The figure shows three views and two pictorial views of one solid part (mm, origin at its lowest corner). Answer the questions. Coordinates: 2 decimals unless noted, no trailing zeros. Order: outer loops, then holes, each group sorted by start corner. A loop starts at its lowest first (then second) coordinate and runs counter-clockwise, first axis right, second up. Notation, with made-up numbers: (-17.75, 46) -> (-9.75, 46) arc R26 ccw to (-9.75, 85) -> close; hole circle Ø8 at (52.25, 67.5). An arc over 180 degrees is marked (long way). Return JSON: item names as keys, results as strings.
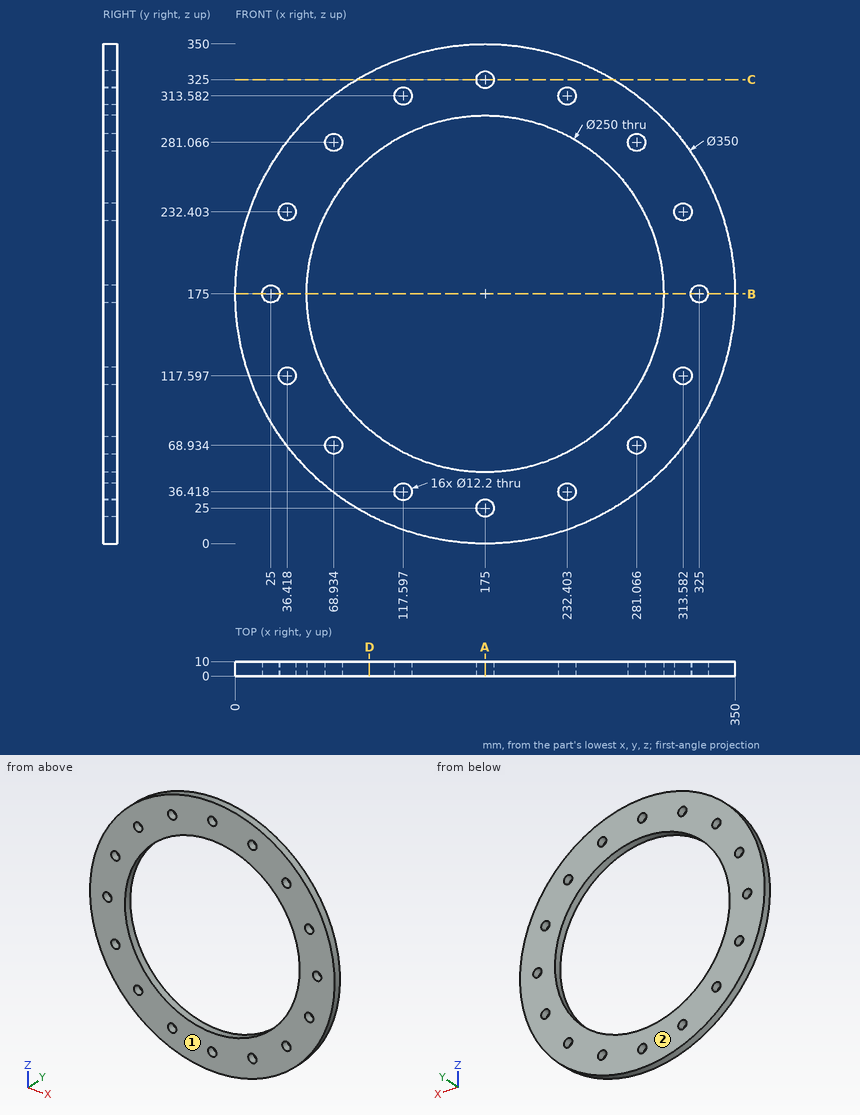
Item 1: Find the intervals of material crossed by probe 1 along X at (y, z) = (6.25, 175); probe 2 along X at (y, z) = (3.5, 170) (1 decimal); probe 3 along Z at (x, y) = (39.5, 6.75) (1 decimal), in increasing order.
Answer list:
{"probe 1": "0 to 18.9, 31.1 to 50, 300 to 318.9, 331.1 to 350", "probe 2": "0.1 to 21.5, 28.5 to 50.1, 299.9 to 321.5, 328.5 to 349.9", "probe 3": "64.3 to 112.3, 122.9 to 227.1, 237.7 to 285.7"}
Item 2: The part is cut by section C-C on z = 325. Determine the outline of the cut face in (x, y), plus the area to 3 significant figures.
Answer list:
{"outline": "(84.86, 0) -> (168.9, 0) -> (168.9, 10) -> (84.86, 10) -> close; (181.1, 0) -> (265.14, 0) -> (265.14, 10) -> (181.1, 10) -> close", "area": "1,680 mm2"}
Item 3: The part is cut by section B-B on z = 175. Determine the outline of the cut face in (x, y).
Answer list:
{"outline": "(0, 0) -> (18.9, 0) -> (18.9, 10) -> (0, 10) -> close; (31.1, 0) -> (50, 0) -> (50, 10) -> (31.1, 10) -> close; (300, 0) -> (318.9, 0) -> (318.9, 10) -> (300, 10) -> close; (331.1, 0) -> (350, 0) -> (350, 10) -> (331.1, 10) -> close"}
Item 4: Flat-ended cylindrical pins translate along their axes: pin 1 (1.5 mm diameter, centred on y = 4, z = 193.5, fed in from -X); pin 2 (5 mm diameter, centred on x = 156, y = 5.5, fed in from +Z); pin 3 (3 mm diameter, centred on y = 5, z = 310, fed in from -X). Find the tip coordinate at first contact, or state that the pin passes through.
Answer list:
{"pin 1": "x = 0.9", "pin 2": "z = 349.22", "pin 3": "x = 61.85"}
Item 5: The part is cut by section A-A on x = 175. Determine the outline of the cut face in (y, z).
Answer list:
{"outline": "(0, 0) -> (10, 0) -> (10, 18.9) -> (0, 18.9) -> close; (0, 31.1) -> (10, 31.1) -> (10, 50) -> (0, 50) -> close; (0, 300) -> (10, 300) -> (10, 318.9) -> (0, 318.9) -> close; (0, 331.1) -> (10, 331.1) -> (10, 350) -> (0, 350) -> close"}
Item 6: Determine the mould class of the marked faces 1 and 2 for opening direction Y: pulls with the +Y half, pulls with the -Y half, needs draft (parallel to the pull), parting line crosses it, or undercut.
Answer list:
{"face 1": "pulls with the -Y half", "face 2": "pulls with the +Y half"}
Item 7: The part is cut by section D-D on x = 94. Determine the outline of the cut face in (y, z) (1 decimal), plus the area to 3 significant figures.
Answer list:
{"outline": "(0, 19.9) -> (10, 19.9) -> (10, 79.8) -> (0, 79.8) -> close; (0, 270.2) -> (10, 270.2) -> (10, 330.1) -> (0, 330.1) -> close", "area": "1,200 mm2"}
